Could you check a few things on this model? Use its own coordinates, in mm. Face numbers are marked on the shaded views. Coordinates: 2 decimals unless noted, no trailing zeros. Order: outer loops, then holes, each group sorted by start corner. A loop starts at its lowest first (then second) coordinate and runs counter-clockwise, first axis right, second up. Notation, with made-up numbers: (12.25, 75) -> (37.25, 75) arc R25 cw to (37.25, 99) -> close; hole circle Ø5 at (-38.75, 42.5). An arc over 180 degrees is marked (long way). Put each result on its own line as item: value. Start each with the question number.
Q1. If we section it at D-D (y = -32): Please give me the cut outline in (x, z), and give its area (3 significant figures).
Q2. Will these pins go through, and if not, where does the flat tip stop? pin 1 (2 mm diameter, centred on x = -32.5, y = -1.5, fed in from -Z); pin 2 (1.6 mm diameter, centred on x = 41, z = 26, fed in from +Y); pin 3 (0.6 mm diameter, centred on x = 24.5, z = 1.5, fed in from -Y); pin 4 (3 mm diameter, centred on x = -25.5, y = 2.5, fed in from +Z).
Q3. If we section it at A-A (z = 17.5): Please give me the cut outline in (x, y), and give its area (3 significant figures).
Q4. We'd pull the mould along X, two halves only. Please class the marked faces 1, 2 and 3: +X half, -X half, draft (parallel to the pull), parting line (faces both ways), or undercut.
Q5. If we section it at C-C (x = -33): Please give me the cut outline in (y, z).
Q6. If we section it at B-B (x = 0): Please give me the cut outline in (y, z), and give its area (3 significant figures).
Q7. Please list where these lines run through material, in increasing order: line 1 along X through (y, z) = (1, 1); line 2 along Y through (x, z) = (-0.5, 3); line 3 along Z through (x, y) = (-31, -9).
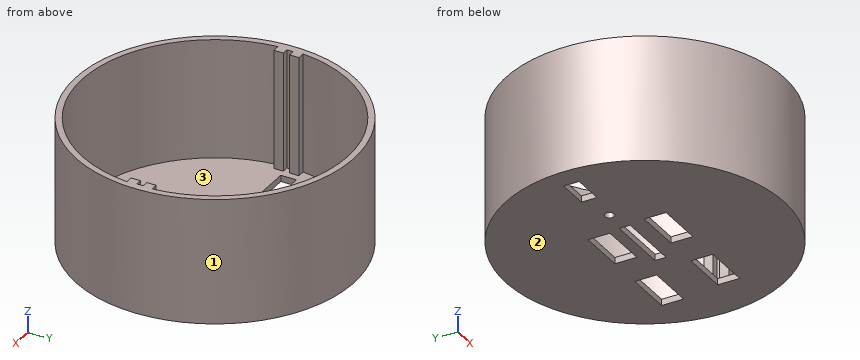
from build123d import *

# Parameters (mm, degrees)
SKETCH_R        = 44.25
PAD_DEPTH       = 40
SKETCH001_R     = 42.25
POCKET_DEPTH    = 38
SKETCH002_W     = 3
SKETCH002_H     = 8
PAD001_DEPTH    = 38
SKETCH003_W     = 3
SKETCH003_H     = 2
POCKET001_DEPTH = 38
SKETCH004_R     = 1.5
SKETCH004_W     = 20
SKETCH004_H     = 3.5
SKETCH004_W_2   = 10
SKETCH004_H_2   = 5
SKETCH004_W_3   = 15
SKETCH004_H_3   = 7
POCKET002_DEPTH = 2


with BuildPart() as part:
    # Sketch → Pad (new body)
    with BuildSketch(Plane.XY):
        Circle(SKETCH_R)
    extrude(amount=PAD_DEPTH)

    # Sketch001 (on Face3 of Pad) → Pocket (cut)
    with BuildSketch(Plane.XY.offset(40)):
        Circle(SKETCH001_R)
    extrude(amount=-POCKET_DEPTH, mode=Mode.SUBTRACT)

    # Sketch002 (on Face5 of Pocket) → Pad001 (join)
    with BuildSketch(Plane.XY.offset(2)):
        with Locations((-41.25, 0)):
            Rectangle(SKETCH002_W, SKETCH002_H)
        with Locations((41.25, 0)):
            Rectangle(SKETCH002_W, SKETCH002_H)
    extrude(amount=PAD001_DEPTH)

    # Sketch003 (on Face14 of Pad001) → Pocket001 (cut)
    with BuildSketch(Plane.XY.offset(40)):
        with Locations((-40.25, 0)):
            Rectangle(SKETCH003_W, SKETCH003_H)
        with Locations((40.25, 0)):
            Rectangle(SKETCH003_W, SKETCH003_H)
    extrude(amount=-POCKET001_DEPTH, mode=Mode.SUBTRACT)

    # Sketch004 (on Face9 of Pocket001) → Pocket002 (cut)
    with BuildSketch(Plane.XY.offset(2)):
        with Locations((-17.5, 1.25)):
            Circle(SKETCH004_R)
        with Locations((0, 0.75)):
            Rectangle(SKETCH004_W, SKETCH004_H)
        with Locations((-32.5, 2)):
            Rectangle(SKETCH004_W_2, SKETCH004_H_2)
        with Locations((-3.5, -9.5)):
            Rectangle(SKETCH004_W_3, SKETCH004_H_3)
        with Locations((22.5, -9.5)):
            Rectangle(SKETCH004_W_3, SKETCH004_H_3)
        with Locations((-1.5, 9.5)):
            Rectangle(SKETCH004_W_3, SKETCH004_H_3)
        with Locations((24.5, 9.5)):
            Rectangle(SKETCH004_W_3, SKETCH004_H_3)
    extrude(amount=-POCKET002_DEPTH, mode=Mode.SUBTRACT)


solid = part.part
The answers:
1. outline: (-30.56, 0) -> (30.56, 0) -> (30.56, 40) -> (27.59, 40) -> (27.59, 2) -> (-27.59, 2) -> (-27.59, 40) -> (-30.56, 40) -> close
1. area: 348 mm^2
2. pin 1: z = 0
2. pin 2: y = 18.49
2. pin 3: y = -37.05
2. pin 4: z = 2
3. outline: circle Ø88.5 at (0, 0); hole (-42.06, -4) arc R42.25 ccw to (42.06, -4) -> (39.75, -4) -> (39.75, -1) -> (41.75, -1) -> (41.75, 1) -> (39.75, 1) -> (39.75, 4) -> (42.06, 4) arc R42.25 ccw to (-42.06, 4) -> (-39.75, 4) -> (-39.75, 1) -> (-41.75, 1) -> (-41.75, -1) -> (-39.75, -1) -> (-39.75, -4) -> close
3. area: 574 mm^2
4. face 1: parting line
4. face 2: draft
4. face 3: undercut
5. outline: (-29.48, 0) -> (-0.5, 0) -> (-0.5, 2) -> (-26.38, 2) -> (-26.38, 40) -> (-29.48, 40) -> close; (4.5, 0) -> (29.48, 0) -> (29.48, 40) -> (26.38, 40) -> (26.38, 2) -> (4.5, 2) -> close
6. outline: (-44.25, 0) -> (-13, 0) -> (-13, 2) -> (-42.25, 2) -> (-42.25, 40) -> (-44.25, 40) -> close; (-6, 0) -> (-1, 0) -> (-1, 2) -> (-6, 2) -> close; (2.5, 0) -> (6, 0) -> (6, 2) -> (2.5, 2) -> close; (13, 0) -> (44.25, 0) -> (44.25, 40) -> (42.25, 40) -> (42.25, 2) -> (13, 2) -> close
6. area: 294 mm^2
7. line 1: -44.24 to -37.5, -27.5 to -18.98, -16.02 to -10, 10 to 44.24
7. line 2: -44.25 to -42.25, 42.25 to 44.25
7. line 3: 0 to 2
